Here's how the part is built. I have some questions about the finished solid (model axes, mm). Coordinates: 2 decimals unless noted, no trailing zeros. Write each loop counter-clockwise with the first axis right and the second up, starting at its lowest first coordinate (ties: lowest second). Pieces come first, ordered by that corner, then holes.
(1) Imagine slicing it at C-C, the plane x = -103.5. List the corners of the cut face in (y, z) for me.
(2) Imagine slicing it at A-A, the plane z = 0.7. List the corners of the cut face in (x, y) for me (3 decimals), plus the area to 3 significant figures.
(3) For pin 1 Ø6 at (x, y) = (-90, 61.5) entering from -Z, with a flat end and sliding along its axis, tell me the tip position at first contact or that it passes through.
(4) Imagine slicing it at B-B, the plane y = 43. List the corners of the cut face in (x, z) for me.
(5) Please list where these lines run through material, in increasing order: probe 1 along X at (y, z) = (62, 0.35); probe 2 along X at (y, z) = (39.5, 0.45); probe 3 along Y at (x, z) = (-85.5, 0.75).
```python
from build123d import *

# Parameters (mm, degrees)
BOSS_EXTRU_1_DEPTH = 2
CONG_1_R           = 10


with BuildPart() as part:
    # Esquisse1 → Boss.-Extru.1 (new body)
    with BuildSketch(Plane.XY):
        Polygon((-99.209210776, 80.763658909), (-55.142491898, 71.646406727), (-65.2727721, 22.683385752), (-109.339490978, 31.800637933), align=None)
    extrude(amount=BOSS_EXTRU_1_DEPTH)

    # Congé1
    cong_1_edges = [part.edges().sort_by_distance(p)[0] for p in [
        (-99.209210776, 80.763658909, 1),
        (-55.142491898, 71.646406727, 1),
        (-65.2727721, 22.683385752, 1),
        (-109.339490978, 31.800637933, 1),
    ]]
    fillet(cong_1_edges, radius=CONG_1_R)


solid = part.part
```
Recorded:
1. outline: (31.55, 0) - (60.02, 0) - (60.02, 2) - (31.55, 2) - close
2. outline: (-107.313, 41.593) arc R10 ccw to (-99.547, 29.775) - (-75.065, 24.709) arc R10 ccw to (-63.247, 32.476) - (-57.169, 61.854) arc R10 ccw to (-64.935, 73.672) - (-89.417, 78.738) arc R10 ccw to (-101.235, 70.971) - close
2. area: 2,160 mm2
3. pin 1: stops at z = 0
4. outline: (-107.02, 0) - (-61.07, 0) - (-61.07, 2) - (-107.02, 2) - close
5. probe 1: x = -103.09 to -57.14
5. probe 2: x = -107.52 to -61.79
5. probe 3: y = 26.87 to 77.93
